Build history of the part. All positions in model axes, mm. A direction names the side the tool comes from. Round coordinates to 2 decimals unless told otherwise and drop trailing zeros. Order: outer loops, then holes, each group sorted by start corner. A loop starts at its lowest first (then second) coordinate and runs counter-clockwise, first axis right, second up. Notation, with made-up numbers: (82.25, 7.5) -> (114.25, 7.5) arc R10 cw to (114.25, 23.5) -> close; hole circle Ø8 at (-26, 26). An arc over 180 degrees is marked (long way). Write item = value, one per line.
from build123d import *

# Parameters (mm, degrees)
SKETCH2_W           = 66.04
SKETCH2_H           = 53.34
BOSS_EXTRUDE1_DEPTH = 1.65
SKETCH3_W           = 15.58
SKETCH3_H           = 11.12
BOSS_EXTRUDE2_DEPTH = 9.75
SKETCH4_W           = 8.3
SKETCH4_H           = 7.204134494
SKETCH4_W_2         = 5.16
SKETCH4_H_2         = 2.74
CUT_EXTRUDE1_DEPTH  = 9.75
SKETCH5_W           = 15.24
SKETCH5_H           = 2.41
SKETCH5_W_2         = 20.32
BOSS_EXTRUDE3_DEPTH = 8.51


with BuildPart() as part:
    # Sketch2 → Boss-Extrude1 (new body)
    with BuildSketch(Plane(origin=(0, 0, 0), x_dir=(1, 0, 0), z_dir=(0, 1, 0))):
        Rectangle(SKETCH2_W, SKETCH2_H)
    extrude(amount=BOSS_EXTRUDE1_DEPTH)

    # Sketch3 → Boss-Extrude2 (add)
    with BuildSketch(Plane(origin=(0, 1.65, 0), x_dir=(1, 0, 0), z_dir=(0, 1, 0))):
        with Locations((-30.66, 9.691373861)):
            Rectangle(SKETCH3_W, SKETCH3_H)
    extrude(amount=BOSS_EXTRUDE2_DEPTH)

    # Sketch4 → Cut-Extrude1 (cut)
    with BuildSketch(Plane.ZY.offset(38.45)):
        with Locations((-9.681373861, 6.202067247)):
            Rectangle(SKETCH4_W, SKETCH4_H)
        with Locations((-9.681373861, 6.202067247)):
            Rectangle(SKETCH4_W_2, SKETCH4_H_2, mode=Mode.SUBTRACT)
    extrude(amount=-CUT_EXTRUDE1_DEPTH, mode=Mode.SUBTRACT)

    # Sketch5 → Boss-Extrude3 (add)
    with BuildSketch(Plane(origin=(0, 1.65, 0), x_dir=(1, 0, 0), z_dir=(0, 1, 0))):
        with Locations((24.13, -24.125)):
            Rectangle(SKETCH5_W, SKETCH5_H)
        with Locations((3.81, -24.125)):
            Rectangle(SKETCH5_W_2, SKETCH5_H)
        with Locations((24.13, 24.125)):
            Rectangle(SKETCH5_W, SKETCH5_H)
        with Locations((3.81, 24.125)):
            Rectangle(SKETCH5_W_2, SKETCH5_H)
    extrude(amount=BOSS_EXTRUDE3_DEPTH)


solid = part.part
Q1. Probe probe 1 along Y at (x, z) = (-35, -12); probe 2 along Z at (x, y) = (-4.5, 5); probe 3 along X at (y, z) = (3.75, -23.5). List the from-to ranges inside material, lowest first.
Check values:
probe_1 = 1.65 to 2.6, 4.83 to 7.57, 9.8 to 11.4
probe_2 = -25.33 to -22.92, 22.92 to 25.33
probe_3 = -6.35 to 13.97, 16.51 to 31.75
Q2. Cut at B-B, the plane x = 17.5. List the corners of the cut face in (y, z).
Check values:
outline = (0, -26.67) -> (1.65, -26.67) -> (1.65, -25.33) -> (10.16, -25.33) -> (10.16, -22.92) -> (1.65, -22.92) -> (1.65, 22.92) -> (10.16, 22.92) -> (10.16, 25.33) -> (1.65, 25.33) -> (1.65, 26.67) -> (0, 26.67) -> close
Q3. Flat gauge pins, fed straight in: pin 1 (4.5 mm diameter, centred on x = -0.5, y = 5.5, fed in from -Z); pin 2 (10 mm diameter, centred on x = -13.5, z = -9, fed in from +Y); pin 3 (1.4 mm diameter, centred on x = -31.5, y = 6, fed in from +Z). Where does each tip first touch, or does it go through?
Check values:
pin_1 = -25.33
pin_2 = 1.65
pin_3 = -4.13
Q4. Cut at D-D, the plane x = -16. List the corners of the cut face in (y, z), and give its area (3 significant figures).
Check values:
outline = (0, -26.67) -> (1.65, -26.67) -> (1.65, 26.67) -> (0, 26.67) -> close
area = 88.0 mm²
Q5. Mould opens along Y. For faces 6 (the face through (13.97, 6, 24)), 7 (the face through (-34, 6, -12.261)), 8 (the face through (24, 10.16, -24)) say: released by +Y, released by -Y, zero draft, split by the parting line, or undercut.
Check values:
face_6 = zero draft
face_7 = undercut
face_8 = released by +Y
Q6. Which spindle directions (+Z, -Z, +X, -X, +Y, -Y) get a long thin tool onto all of the face, cutting with end or side? Do faces 1 (the face through (-31, 6, -4.131)), 2 (the face through (31.75, 6, 24)), 3 (the face through (-34, 6, -7.101)), 4 (the face through (4, 6, -25.33)), 5 (the face through (4, 6, 22.92)). Say none if no direction does.
Check values:
face_1 = +Z, +X, -X, +Y
face_2 = +Z, -Z, +X, +Y
face_3 = -X
face_4 = -Z, +X, -X, +Y
face_5 = +X, -X, +Y
Q7. Cut at A-A, the plane y = 6.25. List the corners of the cut face in (x, z), and give its area (3 significant figures).
Check values:
outline = (-38.45, -15.25) -> (-22.87, -15.25) -> (-22.87, -4.13) -> (-38.45, -4.13) -> (-38.45, -5.53) -> (-28.7, -5.53) -> (-28.7, -7.1) -> (-38.45, -7.1) -> (-38.45, -12.26) -> (-28.7, -12.26) -> (-28.7, -13.83) -> (-38.45, -13.83) -> close; (-6.35, -25.33) -> (13.97, -25.33) -> (13.97, -22.92) -> (-6.35, -22.92) -> close; (-6.35, 22.92) -> (13.97, 22.92) -> (13.97, 25.33) -> (-6.35, 25.33) -> close; (16.51, -25.33) -> (31.75, -25.33) -> (31.75, -22.92) -> (16.51, -22.92) -> close; (16.51, 22.92) -> (31.75, 22.92) -> (31.75, 25.33) -> (16.51, 25.33) -> close
area = 314 mm²
Q8. Cut at C-C, the plane z = 8. List the corners of the cut face in (x, y).
Check values:
outline = (-33.02, 0) -> (33.02, 0) -> (33.02, 1.65) -> (-33.02, 1.65) -> close
